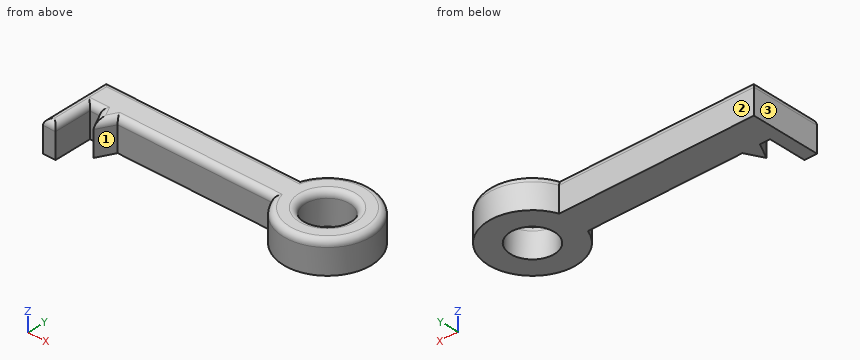
```python
from build123d import *

# Parameters (mm, degrees)
F0_R     = 17.5
F0_W     = 8
F0_H     = 15
F1_DEPTH = 25
F2_R     = 4.99999


# Not quite as in the source:
# - a fillet or chamfer is up to 0.001 mm smaller than in the source, because OpenCascade refuses the exact size


with BuildPart() as f1:
    # F0 (on Top) → F1 (new body)
    with BuildSketch(Plane.XY):
        with BuildLine():
            Line((0, 3.9768594503), (-155, 3.9768594503))
            Line((-155, 3.9768594503), (-155, -21.0231405497))
            Line((-155, -21.0231405497), (-147, -21.0231405497))
            Line((-147, -21.0231405497), (-145, -21.0231405497))
            Line((-145, -21.0231405497), (-137, -21.0231405497))
            Line((-137, -21.0231405497), (-123, -21.0231405497))
            Line((-123, -21.0231405497), (0, -21.0231405497))
            ThreePointArc((0, -21.0231405497), (67.6917420766, -8.5231405497), (0, 3.9768594503))
        make_face()
        with Locations((32.6917420766, -8.5231405497)):
            Circle(F0_R, mode=Mode.SUBTRACT)
        with Locations((-151, -28.5231405497)):
            Rectangle(F0_W, F0_H)
        Polygon((-145, -21.0231405497), (-147, -21.0231405497), (-147, -36.0231405497), (-155, -36.0231405497), (-155, -51.0231405497), (-145, -51.0231405497), align=None)
        Polygon((-130, -34.2896397111), (-123, -21.0231405497), (-137, -21.0231405497), align=None)
    extrude(amount=F1_DEPTH)

    # F2 (radius 5 in the source; OpenCascade refuses exactly that, so slightly less here)
    f2_edges = [f1.edges().sort_by_distance(p)[0] for p in [
        (-77.5, 3.976859, 25),
        (-61.5, -21.023141, 25),
        (-133.5, -27.65639, 25),
        (-155, -23.523141, 25),
        (-145, -36.023141, 25),
        (67.691742, -8.523141, 25),
        (-150, -51.023141, 25),
        (-141, -21.023141, 25),
        (-126.5, -27.65639, 25),
        (15.191742, -8.523141, 25),
    ]]
    fillet(f2_edges, radius=F2_R)


solid = f1.part
```
Here's how the part is built. I have some questions about the finished solid (model axes, mm). Face numbers are marked on the shaded views. A direction names the side the tool comes from. Give positions to 0.01 mm unless a question says otherwise; leave off trailing zeros. Order: outer loops, then holes, each group sorted by start corner. A loop starts at its lowest first (then second) coordinate and runs counter-clockwise, first axis right, second up. Notation, with made-up numbers: (-37.75, -38.75) -> (-1.75, -38.75) arc R3 ccw to (-1.75, -34.75) -> close; hole circle Ø5 at (-19.75, 19). An arc over 180 degrees is marked (long way). Use CSV: the item, a comma, the result in double quotes. Start each with the question number.
Item 1: On a 3-axis mill with a long thin cutter (end or side, diameter ignored), from which of +Z, -Z, +X, -X, +Y, -Y can I reach the whole of each face in a straight line? I mean the marked faces 1, 2 and 3. Say none if no direction works.
Item 2: Suppose I cut it at A-A (x = -34). List the corners of the cut face in (y, z) for me, and give its area (3 significant figures).
Item 3: I'm going to push flat-ended pins straight in: P1, Ø2.5, axis at x = -143, z = 12, coming from the -Y side; P2, Ø6, axis at y = -5, z = 8.5, coming from the +X side; P3, Ø6, axis at y = -21, z = 14.5, coming from the +X side. Where does each tip first touch, or does it pass through?
Item 4: If I drill on probe 1 along X at (y, z) = (-8.5, 8.5); probe 2 along X at (y, z) = (-34, 13.5); probe 3 along Y at (x, z) = (-107.5, 5.25), over which ranges is the centre line in solid material (lowest first)? Write a range as [from, to].
Item 5: Suppose I cut it at B-B (z = 10). List the corners of the cut face in (x, y) for me.
Answer block:
1,face 1,"+Z, -Z, -Y"
1,face 2,"+Z, -Z, -X, +Y"
1,face 3,"+Z, -Z, -X, +Y, -Y"
2,outline,"(-21.02, 0) -> (3.98, 0) -> (3.98, 20) arc R5 ccw to (-1.02, 25) -> (-16.02, 25) arc R5 ccw to (-21.02, 20) -> close"
2,area,"614 mm^2"
3,P1,"stops at y = -21.02"
3,P2,"stops at x = 67.69"
3,P3,"stops at x = 66.38"
4,probe 1,"x = [-155, 15.19], [50.19, 67.69]"
4,probe 2,"x = [-155, -145], [-130.15, -129.85], [8.69, 56.69]"
4,probe 3,"y = [-21.02, 3.98]"
5,outline,"(-155, -51.02) -> (-145, -51.02) -> (-145, -21.02) -> (-137, -21.02) -> (-130, -34.29) -> (-123, -21.02) -> (0, -21.02) arc R35 ccw (long way) to (0, 3.98) -> (-155, 3.98) -> close; hole circle Ø35 at (32.69, -8.52)"
